Verification items for the finished model (mm, model axes). Face numbers are marked on the shaded views. Coordinates: 2 decimals unless noted, no trailing zeros. Order: outer loops, then holes, each group sorted by start corner. A loop starts at its lowest first (then second) coordinate and runs counter-clockwise, first axis right, second up.
Q1. Cross-section at B-B, the plane y = 0. Record the boundary of the cut face in (x, z) (3 decimals).
Q2. Cross-section at A-A, the plane x = -47. Record the boundary of the cut face in (y, z) (3 decimals), and give its area (3 significant figures).
Q3. Cross-section at C-C, the plane z = 196.5. Record the boundary of the cut face in (x, y) (3 decimals).
Q4. Depth check by flat-ended pin: P1, Ø5, axis at y = -45, z = 255.5, coming from the +X side; P2, Ø8, axis at y = 38, z = 237.5, coming from the +X side; P3, Ø2, axis at y = -44, z = 89, coming from the -X side. Enter the tip coordinate at first touch or a pass-through.
Q5. Thickness scan on line 1 (Z direction, x = 0, y = -77) (3 decimals); line 2 (Y direction, x = 2.5, z = 297); line 3 (Y direction, x = -3, z = 283.5). Record the ranges inside material, lowest first.
Q6. Draft check along Y on the marked faces 1 and 2. Enter one of: pulls with the +Y half, pulls with the -Y half, needs draft (parallel to the pull), parting line crosses it, or undercut.
from build123d import *

# Parameters (mm, degrees)
SKETCH1_R                   = 79.375
SKETCH1_R_2                 = 76.2
BOSS_EXTRUDE1_DEPTH         = 320.675
F_4_40_TAPPED_HOLE1_REACH   = 368.517
F_4_40_TAPPED_HOLE1_BORE_R  = 1.1303
F_10_32_TAPPED_HOLE1_REACH  = 368.517
F_10_32_TAPPED_HOLE1_BORE_R = 2.0193
CIRPATTERN1_COUNT           = 6


with BuildPart() as part:
    # Sketch1 → Boss-Extrude1 (new body)
    with BuildSketch(Plane.XY):
        with Locations(Location((0, 0, 0), (0, 0, 180))):
            Circle(SKETCH1_R)
        with Locations(Location((0, 0, 0), (0, 0, 180))):
            Circle(SKETCH1_R_2, mode=Mode.SUBTRACT)
    extrude(amount=BOSS_EXTRUDE1_DEPTH)

    # #4-40 Tapped Hole1 bore → #4-40 Tapped Hole1 (cut, up to next)
    with BuildSketch(Plane(origin=(0, 79.375, 0), x_dir=(1, 0, 0), z_dir=(0, 1, 0)), mode=Mode.PRIVATE) as f_4_40_tapped_hole1_sk1:
        with Locations((0, -79.375)):
            Circle(F_4_40_TAPPED_HOLE1_BORE_R)
    f_4_40_tapped_hole1_tool1 = extrude(f_4_40_tapped_hole1_sk1.sketch, amount=-F_4_40_TAPPED_HOLE1_REACH, mode=Mode.PRIVATE) & part.part
    f_4_40_tapped_hole1 = f_4_40_tapped_hole1_tool1.solids().sort_by_distance((0, 79.375, 79.375))[0]
    add(f_4_40_tapped_hole1, mode=Mode.SUBTRACT)

    # #10-32 Tapped Hole1 bore → #10-32 Tapped Hole1 (cut, up to next)
    with BuildSketch(Plane(origin=(0, 79.375, 0), x_dir=(1, 0, 0), z_dir=(0, 1, 0)), mode=Mode.PRIVATE) as f_10_32_tapped_hole1_sk1:
        with Locations((0, -241.3)):
            Circle(F_10_32_TAPPED_HOLE1_BORE_R)
    f_10_32_tapped_hole1_tool1 = extrude(f_10_32_tapped_hole1_sk1.sketch, amount=-F_10_32_TAPPED_HOLE1_REACH, mode=Mode.PRIVATE) & part.part
    f_10_32_tapped_hole1 = f_10_32_tapped_hole1_tool1.solids().sort_by_distance((0, 79.375, 241.3))[0]
    add(f_10_32_tapped_hole1, mode=Mode.SUBTRACT)

    # CirPattern1: #4-40 Tapped Hole1, #10-32 Tapped Hole1 ×6 about axis
    cirpattern1_axis = Axis((0, 0, 320.675), (0, 0, 1))
    add([f_4_40_tapped_hole1.rotate(cirpattern1_axis, i * 360 / CIRPATTERN1_COUNT) for i in range(1, CIRPATTERN1_COUNT)], mode=Mode.SUBTRACT)
    add([f_10_32_tapped_hole1.rotate(cirpattern1_axis, i * 360 / CIRPATTERN1_COUNT) for i in range(1, CIRPATTERN1_COUNT)], mode=Mode.SUBTRACT)


solid = part.part
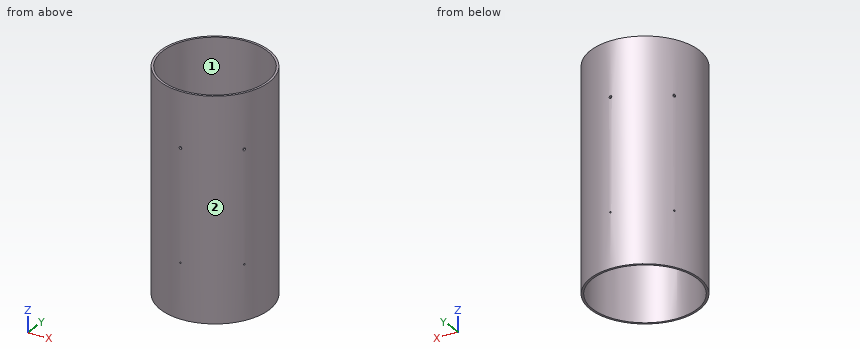
Check values:
1. outline: (-79.375, 0) - (-76.2, 0) - (-76.2, 320.675) - (-79.375, 320.675) - close; (76.2, 0) - (79.375, 0) - (79.375, 320.675) - (76.2, 320.675) - close
2. outline: (-63.964, 0) - (-59.979, 0) - (-59.979, 320.675) - (-63.964, 320.675) - close; (59.979, 0) - (63.964, 0) - (63.964, 320.675) - (59.979, 320.675) - close
2. area: 2,560 mm2
3. outline: circle Ø158.75 at (0, 0); hole circle Ø152.4 at (0, 0)
4. P1: stops at x = 67.04
4. P2: stops at x = 71.72
4. P3: stops at x = -66.72
5. line 1: z = 0 to 78.245, 80.505 to 239.281, 243.319 to 320.675
5. line 2: y = -79.34 to -76.16, 76.16 to 79.34
5. line 3: y = -79.32 to -76.14, 76.14 to 79.32
6. face 1: undercut
6. face 2: parting line crosses it
